Here's how the part is built. I have some questions about the finished solid (model axes, mm). Face numbers are marked on the shaded views. A direction names the side the tool comes from. Round coordinates to 2 decimals unless told otherwise and drop trailing zeros. Order: outer loops, then holes, each group sorted by start corner. A loop starts at its lowest first (then second) coordinate and runs counter-clockwise, first axis right, second up.
```python
from build123d import *

# Parameters (mm, degrees)
CHAMFER1_SIZE = 0.381


with BuildPart() as part:
    # Sketch1 → Revolve1 (revolve)
    with BuildSketch(Plane.XY, mode=Mode.PRIVATE) as revolve1_sk:
        Polygon((-1.778, 1.595281863), (-3.4417, 1.595281863), (-3.4417, -2.976718137), (-4.5085, -2.976718137), (-4.5085, -4.500718137), (-3.9751, -4.500718137), (-3.9751, -19.740718137), (0, -19.740718137), (0, -11.104718137), (-1.778, -11.104718137), align=None)
    revolve(revolve1_sk.sketch.rotate(Axis((0, -11.104718137, 0), (0, 1, 0)), 270), axis=Axis((0, -11.104718137, 0), (0, 1, 0)))

    # Chamfer1
    chamfer1_edges = [part.edges().sort_by_distance(p)[0] for p in [
        (0, 1.595281863, 3.4417),
        (0, 1.595281863, 1.778),
    ]]
    chamfer(chamfer1_edges, length=CHAMFER1_SIZE)


solid = part.part
```
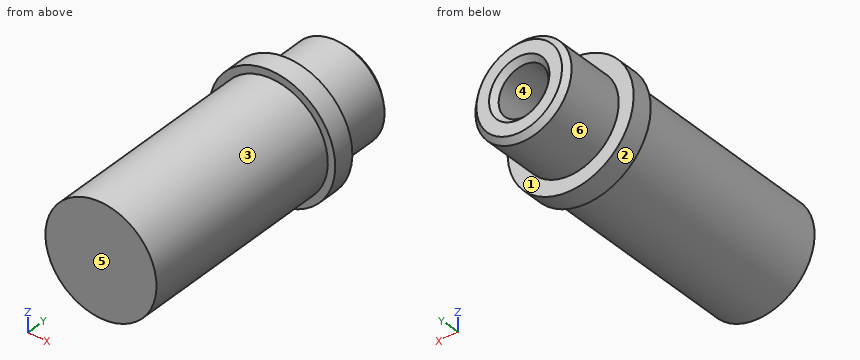
1. I need wall thicknesses on probe 1 along X at (y, z) = (-5.75, 0); probe 2 along Y at (x, z) = (-0.75, 3.75); probe 3 along Y at (x, z) = (2.5, -3.5). Which ranges of each line are inside material? Lowest first, please.
Evaluation:
probe 1: x = -3.98 to -1.78, 1.78 to 3.98
probe 2: y = -19.74 to -2.98
probe 3: y = -4.5 to -2.98
2. If we section it at A-A, the plane z = 0: Write out the boundary of the cut face in (x, y), and give its area (3 significant figures).
Evaluation:
outline: (-4.51, -4.5) - (-3.98, -4.5) - (-3.98, -19.74) - (3.98, -19.74) - (3.98, -4.5) - (4.51, -4.5) - (4.51, -2.98) - (3.44, -2.98) - (3.44, 1.21) - (3.06, 1.6) - (2.16, 1.6) - (1.78, 1.21) - (1.78, -11.1) - (-1.78, -11.1) - (-1.78, 1.21) - (-2.16, 1.6) - (-3.06, 1.6) - (-3.44, 1.21) - (-3.44, -2.98) - (-4.51, -2.98) - close
area: 121 mm2
3. If we mould it in two halves opening along X, with no side actions, what happens to the marked faces 4, 5 and 6? For each: released by +X, released by -X, zero draft, split by the parting line, or undercut.
Evaluation:
face 4: undercut
face 5: zero draft
face 6: split by the parting line
4. If we section it at C-C, the plane y = -8.5: Write out the boundary of the cut face in (x, z).
Evaluation:
outline: circle Ø7.95 at (0, 0); hole circle Ø3.56 at (0, 0)
5. On a 3-axis mill with a long thin cutter (end or side, diameter ignored), from which of +Z, -Z, +X, -X, +Y, -Y can I reach the whole of each face in a straight line? I mean the marked faces 1, 2 and 3. Say none if no direction works.
Evaluation:
face 1: +Y
face 2: +Y, -Y
face 3: -Y
6. If we section it at B-B, the plane x = 0: Write out the boundary of the cut face in (y, z), and give its area (3 significant figures).
Evaluation:
outline: (-19.74, -3.98) - (-4.5, -3.98) - (-4.5, -4.51) - (-2.98, -4.51) - (-2.98, -3.44) - (1.21, -3.44) - (1.6, -3.06) - (1.6, -2.16) - (1.21, -1.78) - (-11.1, -1.78) - (-11.1, 1.78) - (1.21, 1.78) - (1.6, 2.16) - (1.6, 3.06) - (1.21, 3.44) - (-2.98, 3.44) - (-2.98, 4.51) - (-4.5, 4.51) - (-4.5, 3.98) - (-19.74, 3.98) - close
area: 121 mm2
7. I'm going to push flat-ended pins straight in: P1, Ø4, axis at x = 3, z = 2.5, coming from the +Y side; P2, Ø4, axis at y = -13.5, z = -1, coming from the -X side; P3, Ø4, axis at y = -12.5, z = 1, coming from the +X side; P4, Ø2, axis at x = 2.5, y = -9, coming from the +Z side. Where does each tip first touch, or does it pass through?
Evaluation:
P1: stops at y = 1.6
P2: stops at x = -3.98
P3: stops at x = 3.98
P4: stops at z = 3.68
